Verification items for the finished model (mm, model axes). A direction names the side the tool comes from. Give positions to 0.01 mm unless a question says otherwise; leave off trailing zeros. Order: outer loops, then holes, each group sorted by start corner. A loop starts at its lowest first (then second) coordinate and runs counter-clockwise, first axis right, second up. Notation, with made-up numbers: (74, -30.75) - (84, -30.75) arc R26 ccw to (84, 4.25) - close; hole circle Ø6 at (-29, -18.5). An arc over 180 degrees is marked (long way). Answer as a JSON object with one key per item and string values. Group by question number.
(1) Section check A-A (y = -5.5). Record the boundary of the cut face in (x, z), then the cut area to 3 significant figures.
(2) Thickness scan on line 1 (Y direction, x = 18.5, z = 4.4); line 2 (Z direction, x = -1, y = -9.5); line 3 (X direction, y = -13, z = 0.9). Record the ranges inside material, lowest first.
(3) Mould release check, pull along Y, two halves, no side actions. Record for faces 1 (the face through (12.725, 6.848, 5.407)), 2 (the face through (9, 1.111, 5)), 3 (the face through (9, 0, 3.518)), 4 (the face through (-3.484, -13, 1)): +Y half, -Y half, draft (parallel to the pull), parting line (faces both ways), or undercut.
(4) Section check D-D (y = 8.5). Record the boundary of the cut face in (x, z), then the cut area to 3 significant figures.
(5) Section check B-B (x = 11). Record the boundary of the cut face in (y, z).
(6) Section check C-C (z = 5.1). Record the boundary of the cut face in (x, y), then the cut area to 3 significant figures.
(7) Access from +Z, -Z, +X, -X, +Y, -Y to the whole of each face (thin tool, end or side, straight path). Record for faces 5 (the face through (11, 2, 6)), 6 (the face through (12, 9, 3.3)), 7 (the face through (12, -9, 3.3)), 8 (the face through (28.55, 0, 4)), 9 (the face through (-3.484, 13, 1)).
(8) Depth check by flat-ended pin: pin 1 Ø4 at (x, y) = (20.5, 6) entering from +Z; pin 2 Ø2 at (x, z) = (10, 4.5) entering from -Y; pin 3 Ø0.7 at (x, z) = (13.5, 5) entering from -Y. Enter the tip coordinate at first touch or a pass-through.
```python
from build123d import *

# Parameters (mm, degrees)
F0_W      = 57.1
F0_H      = 20
F1_DEPTH  = 3.3
F2_W      = 57.1
F2_H      = 14.253388
F3_DEPTH  = 2.4
F4_R      = 0.976
F5_W      = 2.221158
F5_H      = 4.363652
F6_DEPTH  = 51.4
F7_W      = 54.248591
F7_H      = 2.840603
F8_DEPTH  = 0.3
F9_W      = 1.6
F9_H      = 2
F10_DEPTH = 1.25
F12_DEPTH = 1.25
F13_W     = 20.793454
F13_H     = 7.292897
F14_DEPTH = 25
F15_W     = 32.082847
F15_H     = 32.694116
F16_DEPTH = 1.7


with BuildPart() as f1:
    # F0 (on Top) → F1 (new body)
    with BuildSketch(Plane.XY):
        Rectangle(F0_W, F0_H)
    extrude(amount=F1_DEPTH)

    # F2 (on face) → F3 (join)
    with BuildSketch(Plane.XY.offset(3.3)):
        Rectangle(F2_W, F2_H)
    extrude(amount=F3_DEPTH)

    # F4
    f4_edges = [f1.edges().sort_by_distance(p)[0] for p in [
        (0, -7.126694, 3.3),
        (0, 7.126694, 3.3),
        (0, 7.126694, 5.7),
        (0, -7.126694, 5.7),
    ]]
    fillet(f4_edges, radius=F4_R)

    # F5 (on face) → F6 (cut)
    with BuildSketch(Plane(origin=(-28.55, 0, 0), x_dir=(0, -1, 0), z_dir=(-1, 0, 0))):
        with Locations((0, 5.7)):
            Rectangle(F5_W, F5_H)
    extrude(amount=-F6_DEPTH, mode=Mode.SUBTRACT)

    # F7 (on face) → F8 (join)
    with BuildSketch(Plane.XY.offset(5.7)):
        with Locations((-1.425704, 2.210335)):
            Rectangle(F7_W, F7_H)
        Polygon((25.698591, 3.630636), (-28.55, 3.630636), (-28.55, 1.110579), (-28.55, 0.790033), (25.698591, 0.790033), align=None)
        Polygon((25.698591, -0.790033), (-28.55, -0.790033), (-28.55, -1.110579), (-28.55, -3.630636), (25.698591, -3.630636), align=None)
    extrude(amount=F8_DEPTH)

    # F9 (on face) → F10 (cut)
    with BuildSketch(Plane.XY.offset(6)):
        with Locations((-17.431669, -1.790033)):
            Rectangle(F9_W, F9_H)
    extrude(amount=-F10_DEPTH, mode=Mode.SUBTRACT)

    # F11 (on face) → F12 (cut)
    with BuildSketch(Plane.XY.offset(6)):
        with BuildLine():
            Line((-16.631669, -2.790033), (-18.231669, -2.790033))
            ThreePointArc((-18.231669, -2.790033), (-17.431669, -3.396082), (-16.631669, -2.790033))
        make_face()
    extrude(amount=-F12_DEPTH, mode=Mode.SUBTRACT)

    # F13 (on face) → F14 (cut)
    with BuildSketch(Plane(origin=(-28.55, 0, 0), x_dir=(0, -1, 0), z_dir=(-1, 0, 0))):
        with Locations((0, 2.663676)):
            Rectangle(F13_W, F13_H)
    extrude(amount=-F14_DEPTH, mode=Mode.SUBTRACT)

    # F15 (on Top) → F16 (join)
    with BuildSketch(Plane.XY):
        with Locations((12.557171, 0)):
            Rectangle(F15_W, F15_H)
    extrude(amount=F16_DEPTH)


solid = f1.part
```
Solutions:
{
 "1": {"outline": "(-3.55, 0) - (28.6, 0) - (28.6, 1.7) - (28.55, 1.7) - (28.55, 5.7) - (-3.55, 5.7) - close", "area": "183 mm2"},
 "2": {"line 1": "y = -7.13 to -1.11, 1.11 to 7.13", "line 2": "z = 0 to 3.3", "line 3": "x = -3.48 to 28.6"},
 "3": {"face 1": "+Y half", "face 2": "undercut", "face 3": "undercut", "face 4": "draft"},
 "4": {"outline": "(-3.55, 0) - (28.6, 0) - (28.6, 1.7) - (28.55, 1.7) - (28.55, 3.3) - (-3.55, 3.3) - close", "area": "106 mm2"},
 "5": {"outline": "(-16.35, 0) - (16.35, 0) - (16.35, 1.7) - (10, 1.7) - (10, 3.3) - (8.1, 3.3) arc R0.98 cw to (7.13, 4.28) - (7.13, 4.72) arc R0.98 ccw to (6.15, 5.7) - (3.63, 5.7) - (3.63, 6) - (0.79, 6) - (0.79, 5.7) - (1.11, 5.7) - (1.11, 3.52) - (-1.11, 3.52) - (-1.11, 5.7) - (-0.79, 5.7) - (-0.79, 6) - (-3.63, 6) - (-3.63, 5.7) - (-6.15, 5.7) arc R0.98 ccw to (-7.13, 4.72) - (-7.13, 4.28) arc R0.98 cw to (-8.1, 3.3) - (-10, 3.3) - (-10, 1.7) - (-16.35, 1.7) - close"},
 "6": {"outline": "(-3.55, -7.05) - (28.55, -7.05) - (28.55, 7.05) - (-3.55, 7.05) - (-3.55, 1.11) - (22.85, 1.11) - (22.85, -1.11) - (-3.55, -1.11) - close", "area": "394 mm2"},
 "7": {"face 5": "+Z, +X, -X, +Y, -Y", "face 6": "+Z, +X, -X, +Y", "face 7": "+Z, +X, -X, -Y", "face 8": "+Z, +X, +Y, -Y", "face 9": "+Z, -Z, -X, +Y"},
 "8": {"pin 1": "stops at z = 5.7", "pin 2": "stops at y = -7.51", "pin 3": "stops at y = -7.13"}
}
